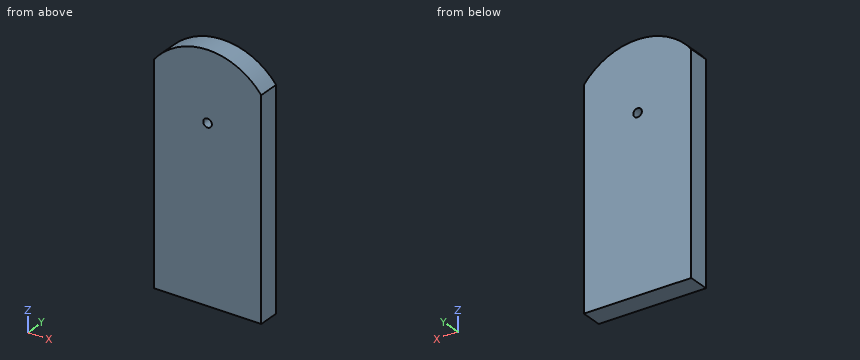
from build123d import *

# Parameters (mm, degrees)
SKETCH1_W           = 50
SKETCH1_H           = 100
SKETCH1_R           = 2
BOSS_EXTRUDE1_DEPTH = 10


with BuildPart() as part:
    # Sketch1 → Boss-Extrude1 (new body)
    # profile 1 of 2: a face of its own
    with BuildSketch(Plane(origin=(0, 0, 0), x_dir=(1, 0, 0), z_dir=(0, 1, 0))):
        Rectangle(SKETCH1_W, SKETCH1_H)
        with Locations(Location((0, -30, 0), (0, 0, 270))):
            Circle(SKETCH1_R, mode=Mode.SUBTRACT)
    # profile 2 of 2: a face of its own
    with BuildSketch(Plane(origin=(0, 0, 0), x_dir=(1, 0, 0), z_dir=(0, 1, 0))):
        with BuildLine():
            Line((-25, -50), (25, -50))
            ThreePointArc((25, -50), (0, -62.015621187), (-25, -50))
        make_face()
    extrude(amount=BOSS_EXTRUDE1_DEPTH)


solid = part.part
Can you work these out from the model? Positions are in its coordinate system, mm. Give positions to 0.01 mm unless a question says otherwise; leave off trailing zeros. Order: outer loops, then holes, each group sorted by start corner. A loop starts at its lowest first (then second) coordinate and runs counter-clockwise, first axis right, second up. Notation, with made-up numbers: M 1,-3.5 L 12,-3.5 A20 ccw 12,8.5 Z; hole C 66.5,27 d3. An arc over 180 degrees is marked long. One line per item, written item: value.
Item 1: Please list where these lines run through material, in increasing order: line 1 (X direction, y = 6, z = 30); line 2 (X direction, y = 5.75, z = 29); line 3 (Z direction, x = -14, y = 8.25).
Verdict:
line 1: -25 to -2, 2 to 25
line 2: -25 to -1.73, 1.73 to 25
line 3: -50 to 58.79
Item 2: If we section it at C-C on y = 6.75: Write out the boundary of the cut face in (x, z).
Verdict:
outline: M -25,-50 L 25,-50 L 25,50 A32.02 ccw -25,50 Z; hole C 0,30 d4
Item 3: If we section it at D-D on x = 15.5: Write out the boundary of the cut face in (y, z), and give its area (3 significant figures).
Verdict:
outline: M 0,-50 L 10,-50 L 10,58.01 L 0,58.01 Z
area: 1,080 mm2
Item 4: For pin 1 (1 mm diameter, centred on x = 16, z = 15.5, fed in from -Y), with a flat end and sliding along its axis, tell me the tip position at first contact or that it passes through.
Verdict:
pin 1: y = 0
Item 5: If we section it at A-A on z = 30: Write out the boundary of the cut face in (x, y), and give its area (3 significant figures).
Verdict:
outline: M -25,0 L -2,0 L -2,10 L -25,10 Z; M 2,0 L 25,0 L 25,10 L 2,10 Z
area: 460 mm2
Item 6: If we section it at B-B on x = 0: Write out the boundary of the cut face in (y, z).
Verdict:
outline: M 0,-50 L 10,-50 L 10,28 L 0,28 Z; M 0,32 L 10,32 L 10,62.02 L 0,62.02 Z
